Source: CAD feature listing. Evaluate the final solid. Frame: model axes, mm. Give positions to 0.01 mm unless a question says otherwise; leave off trailing zeros. Order: outer loops, then holes, each group sorted by start corner. A loop starts at its lowest first (then second) coordinate and runs counter-clockwise, first axis right, second up.
from build123d import *

# Parameters (mm, degrees)
SKETCH2_R           = 26.799999994
BOSS_EXTRUDE1_DEPTH = 3.175
SKETCH3_W           = 3.81
SKETCH3_H           = 3.81
SKETCH3_R           = 1.25
CUT_EXTRUDE1_DEPTH  = 3.175
SKETCH4_R           = 5.5
CUT_EXTRUDE2_DEPTH  = 7.62
CUT_EXTRUDE3_DEPTH  = 5.08


with BuildPart() as part:
    # Sketch2 → Boss-Extrude1 (new body)
    with BuildSketch(Plane(origin=(0, 0, 0), x_dir=(1, 0, 0), z_dir=(0, 1, 0))):
        with Locations(Location((0, 0, 0), (0, 0, 270))):
            Circle(SKETCH2_R)
    extrude(amount=BOSS_EXTRUDE1_DEPTH)

    # Sketch3 → Cut-Extrude1 (cut)
    with BuildSketch(Plane(origin=(0, 3.175, 0), x_dir=(1, 0, 0), z_dir=(0, 1, 0))):
        with Locations((-5e-05, 19.3675)):
            Rectangle(SKETCH3_W, SKETCH3_H)
        with BuildLine():
            ThreePointArc((-1.90505, 21.2725), (-5e-05, 23.1775), (1.90495, 21.2725))
            Line((1.90495, 21.2725), (-1.90505, 21.2725))
        make_face()
        with BuildLine():
            Line((-1.90505, 17.4625), (1.90495, 17.4625))
            ThreePointArc((1.90495, 17.4625), (-5e-05, 15.5575), (-1.90505, 17.4625))
        make_face()
        Polygon((16.0810614, -7.084700603), (19.374239178, -9.000706899), (17.458232881, -12.293884676), (14.165055104, -10.37787838), align=None)
        with BuildLine():
            ThreePointArc((14.165055104, -10.37787838), (13.476469363, -7.773286343), (16.0810614, -7.084700603))
            Line((16.0810614, -7.084700603), (14.165055104, -10.37787838))
        make_face()
        with BuildLine():
            Line((17.458232881, -12.293884676), (19.374239178, -9.000706899))
            ThreePointArc((19.374239178, -9.000706899), (20.062824918, -11.605298935), (17.458232881, -12.293884676))
        make_face()
        Polygon((-14.170405114, -10.381138379), (-16.075405114, -7.081581591), (-19.374961902, -8.986581591), (-17.469961902, -12.286138379), align=None)
        with BuildLine():
            Line((-14.170405114, -10.381138379), (-16.075405114, -7.081581591))
            ThreePointArc((-16.075405114, -7.081581591), (-13.473126719, -7.778859985), (-14.170405114, -10.381138379))
        make_face()
        with BuildLine():
            Line((-17.469961902, -12.286138379), (-19.374961902, -8.986581591))
            ThreePointArc((-19.374961902, -8.986581591), (-20.072240296, -11.588859985), (-17.469961902, -12.286138379))
        make_face()
        with Locations(Location((-10.998522628, -6.35, 0), (0, 0, 270))):
            Circle(SKETCH3_R)
        with Locations(Location((0, 12.7, 0), (0, 0, 270))):
            Circle(SKETCH3_R)
        with Locations(Location((10.998522628, -6.35, 0), (0, 0, 270))):
            Circle(SKETCH3_R)
    extrude(amount=-CUT_EXTRUDE1_DEPTH, mode=Mode.SUBTRACT)

    # Sketch4 → Cut-Extrude2 (cut)
    with BuildSketch(Plane(origin=(0, 3.175, 0), x_dir=(1, 0, 0), z_dir=(0, 1, 0))):
        with Locations(Location((10.998522628, 6.35, 0), (0, 0, 270))):
            Circle(SKETCH4_R)
    extrude(amount=-CUT_EXTRUDE2_DEPTH, mode=Mode.SUBTRACT)

    # Sketch5 → Cut-Extrude3 (cut)
    with BuildSketch(Plane(origin=(0, 3.175, 0), x_dir=(1, 0, 0), z_dir=(0, 1, 0))):
        Polygon((-4.216675415, -24.431543942), (1.41248971, -21.181543942), (-4.93751029, -10.183021314), (-10.566675415, -13.433021314), align=None)
        Polygon((-15.222067079, 0.010353577), (-13.022362553, 1.280353577), (-18.102362553, 10.079171679), (-20.302067079, 8.809171679), align=None)
    extrude(amount=-CUT_EXTRUDE3_DEPTH, mode=Mode.SUBTRACT)


solid = part.part
1) Ray query, L1, parallel to X at y = 2.45, z = 8; L2, parallel to Z at x = -19.5, y = 1.5; L3, parallel to X at y = 2.6, z = -5.5. Return the intervals inside material, ascending.
Checks:
L1: x = -25.58 to -17.67, -13.36 to 13.36, 17.65 to 25.58
L2: z = -18.38 to -9.27, -7.42 to 9.07, 12.21 to 18.38
L3: x = -26.23 to -18.39, -15.46 to 5.56, 16.43 to 26.23
2) First-contact query: pin 1 Ø2 at (x, z) = (0, -12.7) entering from -Y; pin 2 Ø1 at (y, z) = (1.5, -2) entering from +X; pin 3 Ø1.6 at (y, z) = (1.5, -19.5) entering from +X. Flat tips, straight axial feed; report the tip coordinate or a pass-through.
Checks:
pin 1: passes through
pin 2: stops at x = 26.76
pin 3: stops at x = 19.2
3) Section query A-A on z = -6.35. Output: boundary loops of the cut face in (x, y) (3 decimals).
Checks:
outline: (-26.037, 0) - (-18.882, 0) - (-18.882, 3.175) - (-26.037, 3.175) - close; (-15.949, 0) - (5.499, 0) - (5.499, 3.175) - (-15.949, 3.175) - close; (16.499, 0) - (26.037, 0) - (26.037, 3.175) - (16.499, 3.175) - close
4) Section query C-C on z = -18.5. Output: boundary loops of the cut face in (x, y) (3 decimals), and give its area (3 significant figures).
Checks:
outline: (-19.39, 0) - (-1.905, 0) - (-1.905, 3.175) - (-19.39, 3.175) - close; (1.905, 0) - (19.39, 0) - (19.39, 3.175) - (1.905, 3.175) - close
area: 111 mm2
5) Section query B-B on x = 9. Output: boundary loops of the cut face in (y, z) (3 decimals).
Checks:
outline: (0, -25.244) - (3.175, -25.244) - (3.175, -11.474) - (0, -11.474) - close; (0, -1.226) - (3.175, -1.226) - (3.175, 25.244) - (0, 25.244) - close
6) Pull-direction query (X, two-part tool) for faces 1 (the face through (26.57, 1.57, -3.49)), 2 (the face through (0, 3.175, 0)), 3 (the face through (-1.718, 1.61, 15.759)); classes: +X half, -X half, draft (parallel to the pull), parting line (faces both ways), or undercut.
Checks:
face 1: parting line
face 2: draft
face 3: undercut
7) Section query D-D on y = 1.6. State how many separate pieces and enclosed holes the cut face has, and give its area (3 significant figures).
Checks:
separate pieces: 1
enclosed holes: 9
area: 1,960 mm2
